Check sheet for the modelled part. Datum: model origin and axes. Units: mm. Face numbers are marked on the shaded views. A direction names the side the tool comes from. Give positions to 0.01 mm unless a question says otherwise; leave off trailing zeros. Order: outer loops, then holes, each group sorted by start corner. A loop starts at its lowest first (then second) coordinate and runs counter-clockwise, first axis right, second up.
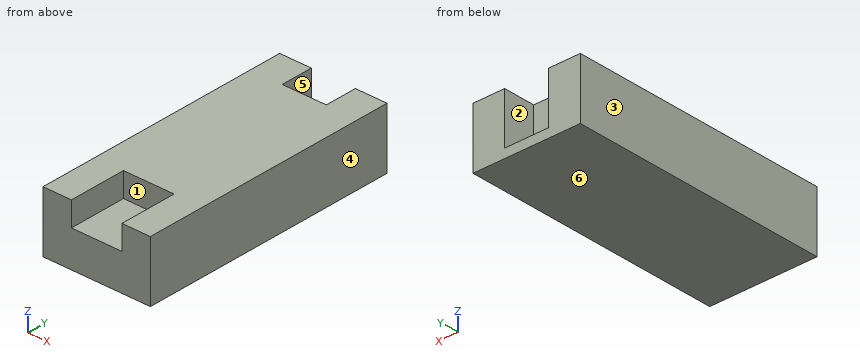
from build123d import *

# Parameters (mm, degrees)
F0_W     = 17.78
F0_H     = 43.18
F1_DEPTH = 1.5
F3_DEPTH = 8.5
F4_DEPTH = 4.5


with BuildPart() as f1:
    # F0 (on Top) → F1 (new body)
    with BuildSketch(Plane.XY):
        Rectangle(F0_W, F0_H)
    extrude(amount=F1_DEPTH)

    # F2 (on face) → F3 (join)
    with BuildSketch(Plane.XY.offset(1.5)):
        Polygon((-3.65, 16.29), (-3.65, 21.59), (-8.89, 21.59), (-8.89, -21.59), (-4.19, -21.59), (-4.19, -12.09), (4.19, -12.09), (4.19, -21.59), (8.89, -21.59), (8.89, 21.59), (3.65, 21.59), (3.65, 16.29), align=None)
    extrude(amount=F3_DEPTH)

    # F4 (add): a face of the model
    f4_faces = [f1.faces().sort_by_distance(p)[0] for p in [
        (0, -16.84, 1.5),
    ]]
    extrude(f4_faces, amount=F4_DEPTH)


solid = f1.part
1) Set-up check for the marked faces 1, 2 and 3: record each of +Z, -Z, +X, -X, +Y, -Y from which the full face is reachable in a straight line by a thin tool's end or side.
Recorded:
face 1: +Z, -Y
face 2: +Z, +Y
face 3: +Z, -Z, -X, +Y, -Y
2) Draft check along X on the marked faces 4, 5 and 6. Enter one of: +X half, -X half, draft (parallel to the pull), parting line (faces both ways), or undercut.
Recorded:
face 4: +X half
face 5: undercut
face 6: draft
3) Material ranges on L1, parallel to X at y = -15, z = 8.25; L2, parallel to Y at x = 1.25, z = 8.75; L3, parallel to Z at x = -2.5, y = -15, recorded low to high.
Recorded:
L1: x = -8.89 to -4.19, 4.19 to 8.89
L2: y = -12.09 to 16.29
L3: z = 0 to 6
4) Depth check by flat-ended pin: pin 1 Ø2 at (x, z) = (0.5, 7.5) entering from -Y; pin 2 Ø1.6 at (x, y) = (-1, 19) entering from +Z. Enter the tip coordinate at first touch or a pass-through.
Recorded:
pin 1: stops at y = -12.09
pin 2: stops at z = 1.5
5) Section check B-B, the plane y = -16. Record the cut outline in (x, z), then the cut area to 3 significant figures.
Recorded:
outline: (-8.89, 0) - (8.89, 0) - (8.89, 10) - (4.19, 10) - (4.19, 6) - (-4.19, 6) - (-4.19, 10) - (-8.89, 10) - close
area: 144 mm2
6) Section check C-C, the plane z = 6.75. Record the cut outline in (x, y).
Recorded:
outline: (-8.89, -21.59) - (-4.19, -21.59) - (-4.19, -12.09) - (4.19, -12.09) - (4.19, -21.59) - (8.89, -21.59) - (8.89, 21.59) - (3.65, 21.59) - (3.65, 16.29) - (-3.65, 16.29) - (-3.65, 21.59) - (-8.89, 21.59) - close
7) Section check A-A, the plane x = 1.75. Record the cut outline in (y, z).
Recorded:
outline: (-21.59, 0) - (21.59, 0) - (21.59, 1.5) - (16.29, 1.5) - (16.29, 10) - (-12.09, 10) - (-12.09, 6) - (-21.59, 6) - close
